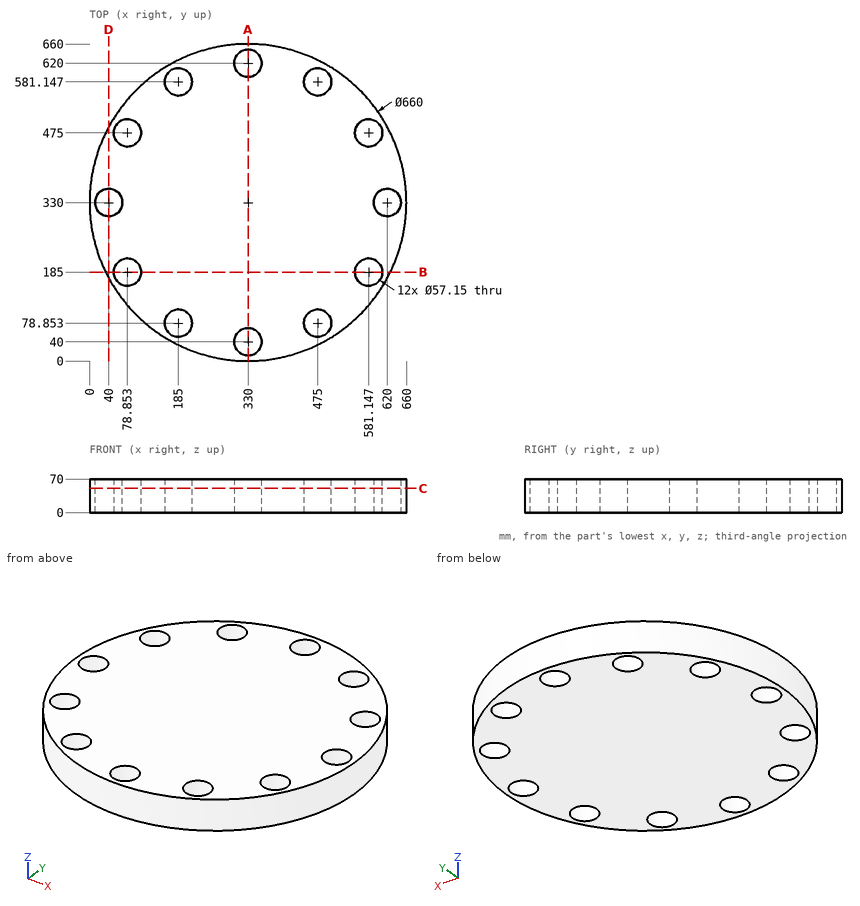
For this review, use the dimensioned drawing (mm, ordinates from the lowest corner) and the shaded views. Coordinates: 2 decimals unless noted, no trailing zeros. Loops run counter-clockwise (first coordinate to the right, second up) from the corner with the lowest first, then second, coordinate; pieces in that order, holes last. Notation, with made-up numbers: (-21.5, -16.5) - (-6.5, -16.5) arc R27 ccw to (-6.5, 13.5) - close; hole circle Ø4 at (86, 59). An arc over 180 degrees is marked (long way). Use one line per item in the form item = value. Start each with the question number.
1) Take a section at C-C (z = 50.5). State how many separate pieces and enclosed holes the cut face has, plus the area to 3 significant figures.
2) Take a section at A-A (x = 330). State the section outline as (y, z) points (1 decimal).
3) Take a section at D-D (x = 40). State the section outline as (y, z) points (1 decimal), plus the area to 3 significant figures.
4) To check wall thickness, follow probe 1 along Y at (x, z) = (330, 21) (1 decimal); probe 2 along X at (y, z) = (185, 41); probe 3 along X at (y, z) = (179, 4) (1 decimal). State the ranges of each line that lie inside material, in increasing order. Write a range as from..to.
5) Take a section at B-B (y = 185). State the section outline as (x, z) points, plus the area to 3 significant figures.
6) For pin 1 (4 mm diameter, centred on x = 504, z = 14.5, fed in from -Y); pin 2 (3 mm diameter, centred on y = 458, z = 17, fed in from +X); pin 3 (3 mm diameter, centred on x = 270, y = 289.5, fed in from -Z); pin 4 (4 mm diameter, centred on x = 169.5, z = 21.5, fed in from -Y), all flat-tipped, find the tip position at first contact; note any pin that passes through.
From the geometry:
q1.separate_pieces = 1
q1.enclosed_holes = 12
q1.area = 311,000 mm2
q2.outline = (0, 0) - (11.4, 0) - (11.4, 70) - (0, 70) - close; (68.6, 0) - (591.4, 0) - (591.4, 70) - (68.6, 70) - close; (648.6, 0) - (660, 0) - (660, 70) - (648.6, 70) - close
q3.outline = (172.5, 0) - (301.4, 0) - (301.4, 70) - (172.5, 70) - close; (358.6, 0) - (487.5, 0) - (487.5, 70) - (358.6, 70) - close
q3.area = 18,000 mm2
q4.probe_1 = 0..11.4, 68.6..591.4, 648.6..660
q4.probe_2 = 33.56..50.28, 107.43..552.57, 609.72..626.44
q4.probe_3 = 36.6..50.9, 106.8..553.2, 609.1..623.4
q5.outline = (33.56, 0) - (50.28, 0) - (50.28, 70) - (33.56, 70) - close; (107.43, 0) - (552.57, 0) - (552.57, 70) - (107.43, 70) - close; (609.72, 0) - (626.44, 0) - (626.44, 70) - (609.72, 70) - close
q5.area = 33,500 mm2
q6.pin_1 = 48.37
q6.pin_2 = 634.79
q6.pin_3 = 0
q6.pin_4 = 40.56
